The listing builds one solid part. Answer for the finished solid, in the listing's coordinates (mm). A direction names the side the tool comes from. Coordinates: 2 decimals unless noted, no trailing zeros. Order: outer loops, then holes, each group sorted by start corner. A loop starts at its lowest first (then second) coordinate and runs counter-clockwise, first axis right, second up. Notation, with made-up numbers: (-34.75, 65.25) - (0.25, 65.25) arc R16 cw to (0.25, 71.25) - close; hole circle Ø11 at (-24.75, -13.75). An arc over 180 degrees is marked (long way). One line per item, written item: value. Start each with the question number.
```python
from build123d import *

# Parameters (mm, degrees)
SKETCH_1_R      = 1.6
SKETCH_1_W      = 14.377962021
SKETCH_1_H      = 2
EXTRUDE_1_DEPTH = 2


with BuildPart() as part:
    # 草图1 → 凸台-拉伸1 (new body)
    with BuildSketch(Plane.XY):
        with BuildLine():
            Line((68, 1), (70, 1))
            Line((70, 1), (66, 5))
            Line((66, 5), (0.546713687, 8.983379328))
            ThreePointArc((0.546713687, 8.983379328), (-9, 0), (0.546713687, -8.983379328))
            Line((0.546713687, -8.983379328), (66, -5))
            Line((66, -5), (70, -1))
            Line((70, -1), (68, -1))
            Line((68, -1), (68, 1))
        make_face()
        Circle(SKETCH_1_R, mode=Mode.SUBTRACT)
        Polygon((30, 1.05), (28.6, 1.05), (28.6, 3.15), (25.5, 3.15), (25.5, 1.05), (21.5, 1.05), (21.5, -1.05), (30, -1.05), align=None, mode=Mode.SUBTRACT)
        Polygon((8.317846196, 4.101632549), (19.58225642, 3.420369402), (19.58225642, -3.420369402), (8.317846196, -4.101632549), align=None, mode=Mode.SUBTRACT)
        with Locations((57.811018989, 0)):
            Rectangle(SKETCH_1_W, SKETCH_1_H, mode=Mode.SUBTRACT)
        Polygon((47.752262622, -2.05), (35.993942407, -2.669181187), (34.25663283, -1.05), (32.998759736, -1.05), (32.998759736, 1.05), (34.25663283, 1.05), (35.993942407, 2.669181187), (47.752262622, 2.05), align=None, mode=Mode.SUBTRACT)
    extrude(amount=EXTRUDE_1_DEPTH)


solid = part.part
```
(1) The part is cut by section D-D on x = 44. Determine the outline of the cut face in (y, z).
(2) Consider probe 1 along X at (y, z) = (-0.25, 1.45); probe 2 along Y at (x, z) = (0, 1.55); probe 3 along X at (y, z) = (2.75, 1). Determine where each line is inside the solid, lowest interval first.
(3) Flat-ended cylindrical pins translate along their axes: pin 1 Ø0.6 at (y, z) = (0, 1) entering from +X; pin 2 Ø0.6 at (x, z) = (25, 0.5) entering from +Y; pin 3 Ø0.6 at (x, z) = (23, 1) entering from -Y. Find the tip coordinate at first contact, or state that the pin passes through.
(4) The part is cut by section B-B on z = 1.5. Count the separate pieces of the cut face and the enclosed holes in it, plus the area to 3 significant figures.
(5) The part is cut by section C-C on x = 57.5. Determine the outline of the cut face in (y, z), plus the area to 3 significant figures.
(6) The part is cut by section A-A on y = 0. Determine the outline of the cut face in (x, z), plus the area to 3 significant figures.
(7) For faces 1 (the face through (69, 1, 1)), 2 (the face through (25.5, 2, 1)), 3 (the face through (33.732, 6.964, 0.986)), determine the directions among +Z, -Z, +X, -X, +Y, -Y from which every point of the face is accessible in a straight line to the end or side of a thin tool.
Completed:
1. outline: (-6.34, 0) - (-2.25, 0) - (-2.25, 2) - (-6.34, 2) - close; (2.25, 0) - (6.34, 0) - (6.34, 2) - (2.25, 2) - close
2. probe 1: x = -9 to -1.58, 1.58 to 8.32, 19.58 to 21.5, 30 to 33, 47.75 to 50.62, 65 to 68
2. probe 2: y = -9 to -1.6, 1.6 to 9
2. probe 3: x = -8.57 to 8.32, 19.58 to 25.5, 28.6 to 68.25
3. pin 1: stops at x = 68
3. pin 2: stops at y = 7.51
3. pin 3: stops at y = -7.64
4. separate pieces: 1
4. enclosed holes: 5
4. area: 862 mm2
5. outline: (-5.52, 0) - (-1, 0) - (-1, 2) - (-5.52, 2) - close; (1, 0) - (5.52, 0) - (5.52, 2) - (1, 2) - close
5. area: 18.1 mm2
6. outline: (-9, 0) - (-1.6, 0) - (-1.6, 2) - (-9, 2) - close; (1.6, 0) - (8.32, 0) - (8.32, 2) - (1.6, 2) - close; (19.58, 0) - (21.5, 0) - (21.5, 2) - (19.58, 2) - close; (30, 0) - (33, 0) - (33, 2) - (30, 2) - close; (47.75, 0) - (50.62, 0) - (50.62, 2) - (47.75, 2) - close; (65, 0) - (68, 0) - (68, 2) - (65, 2) - close
6. area: 49.8 mm2
7. face 1: +Z, -Z, +X
7. face 2: +Z, -Z
7. face 3: +Z, -Z, +X, +Y
